from build123d import *

# Parameters (mm, degrees)
PAD_DEPTH       = 2
BOX002_W        = 44
BOX002_H        = 17
BOX002_DEPTH    = 78
SKETCH003_R     = 4.1
SKETCH003_R_2   = 2
SKETCH003_W     = 49.28004
SKETCH003_H     = 11.88092
POCKET003_DEPTH = 17.001
BOX001_W        = 65
BOX001_H        = 34
BOX001_DEPTH    = 5
BOX_W           = 5
BOX_H           = 34
BOX_DEPTH       = 46
SKETCH_R        = 2.05
POCKET_DEPTH    = 5
SKETCH001_R     = 5
SKETCH001_R_2   = 1.7
POCKET001_DEPTH = 5
SKETCH002_R     = 4.5
POCKET002_DEPTH = 5
SKETCH007_R     = 11.05
POCKET004_DEPTH = 17.001
SKETCH008_R     = 12
SKETCH008_R_2   = 10
PAD001_DEPTH    = 2
CHAMFER_SIZE    = 1
CHAMFER001_SIZE = 1.999


with BuildPart() as pad:
    # Sketch006 → Pad (new body)
    with BuildSketch(Plane.XZ.offset(2)):
        Polygon((-30, 51), (35, 51), (35, 46), (5, 0), (0, 0), (-30, 46), align=None)
    extrude(amount=PAD_DEPTH)


with BuildPart() as pocket003:
    # Box002 → Box002 (new body)
    with BuildSketch(Plane(origin=(-19.5, 15, 51), x_dir=(1, 0, 0), z_dir=(0, 0, 1))):
        with Locations((22, 8.5)):
            Rectangle(BOX002_W, BOX002_H)
    extrude(amount=BOX002_DEPTH)

    # Sketch003 → Pocket003 (cut, through all)
    with BuildSketch(Plane(origin=(-19.5, 15, 51), x_dir=(1, 0, 0), z_dir=(0, -1, 0))):
        with Locations((22, 6)):
            Circle(SKETCH003_R)
        with Locations((22, 63)):
            Circle(SKETCH003_R)
        with Locations((6.95, 19.45)):
            Circle(SKETCH003_R_2)
        with Locations((37.05, 19.45)):
            Circle(SKETCH003_R_2)
        with Locations((6.95, 49.55)):
            Circle(SKETCH003_R_2)
        with Locations((37.05, 49.55)):
            Circle(SKETCH003_R_2)
        with Locations((21.985447, 75.94046)):
            Rectangle(SKETCH003_W, SKETCH003_H)
    extrude(amount=-POCKET003_DEPTH, mode=Mode.SUBTRACT)


with BuildPart() as cubo001:
    # Box001 → Box001 (new body)
    with BuildSketch(Plane(origin=(-30, -2, 46), x_dir=(1, 0, 0), z_dir=(0, 0, 1))):
        with Locations((32.5, 17)):
            Rectangle(BOX001_W, BOX001_H)
    extrude(amount=BOX001_DEPTH)


with BuildPart() as chamfer001:
    # Box → Box (new body)
    with BuildSketch(Plane(origin=(0, -2, 0), x_dir=(1, 0, 0), z_dir=(0, 0, 1))):
        with Locations((2.5, 17)):
            Rectangle(BOX_W, BOX_H)
    extrude(amount=BOX_DEPTH)

    # Fusion: union Cubo001
    add(cubo001.part)

    # Sketch → Pocket (cut)
    with BuildSketch(Plane.XY.offset(51)):
        with Locations((-36.05, -7.05)):
            Circle(SKETCH_R)
        with Locations((28.95, 3.05)):
            Circle(SKETCH_R)
        with Locations((-55.15, -7.05)):
            Circle(SKETCH_R)
        with Locations((9.85, 3.05)):
            Circle(SKETCH_R)
        with Locations((-4.85, 3.05)):
            Circle(SKETCH_R)
        with Locations((-23.95, 3.05)):
            Circle(SKETCH_R)
        with Locations((-23.95, 26.95)):
            Circle(SKETCH_R)
        with Locations((-4.85, 26.95)):
            Circle(SKETCH_R)
        with Locations((9.85, 26.95)):
            Circle(SKETCH_R)
        with Locations((28.95, 26.95)):
            Circle(SKETCH_R)
    extrude(amount=-POCKET_DEPTH, mode=Mode.SUBTRACT)

    # Sketch001 → Pocket001 (cut)
    with BuildSketch(Plane.YZ.offset(5)):
        with Locations((15, 11)):
            Circle(SKETCH001_R)
        with Locations((15, 19.2)):
            Circle(SKETCH001_R_2)
        with Locations((23.2, 11)):
            Circle(SKETCH001_R_2)
        with Locations((15, 2.8)):
            Circle(SKETCH001_R_2)
        with Locations((6.8, 11)):
            Circle(SKETCH001_R_2)
    extrude(amount=-POCKET001_DEPTH, mode=Mode.SUBTRACT)

    # Sketch002 → Pocket002 (cut)
    with BuildSketch(Plane.YZ.offset(5)):
        with Locations((15, 34.8)):
            Circle(SKETCH002_R)
    extrude(amount=-POCKET002_DEPTH, mode=Mode.SUBTRACT)

    # Fusion001: union Pad, Pocket003
    add(pad.part)
    add(pocket003.part)

    # Sketch007 → Pocket004 (cut, through all)
    with BuildSketch(Plane.XZ.offset(-15)):
        with Locations((3.631613, 115.011309)):
            Circle(SKETCH007_R)
    extrude(amount=-POCKET004_DEPTH, mode=Mode.SUBTRACT)

    # Sketch008 → Pad001 (new body)
    with BuildSketch(Plane.XZ.offset(-15)):
        with Locations((2.5, 85.5)):
            Circle(SKETCH008_R)
        with Locations((2.5, 85.5)):
            Circle(SKETCH008_R_2, mode=Mode.SUBTRACT)
    extrude(amount=PAD001_DEPTH)

    # Chamfer
    chamfer_edges = [chamfer001.edges().sort_by_distance(p)[0] for p in [
        (-30, 32, 48.5),
    ]]
    chamfer(chamfer_edges, length=CHAMFER_SIZE)

    # Chamfer001
    chamfer001_edges = [chamfer001.edges().sort_by_distance(p)[0] for p in [
        (24.5, 32, 86),
    ]]
    chamfer(chamfer001_edges, length=CHAMFER001_SIZE)


solid = chamfer001.part
Can you work these out from the model? Positions are in its coordinate system, mm. A direction names the side the tool comes from. Give positions to 0.01 mm unless a question says otherwise; leave off trailing zeros. Loops run counter-clockwise (first coordinate to the right, second up) from the corner with the lowest first, then second, coordinate; pieces in that order, holes last. Notation, with made-up numbers: M 19,3 L 74,3 A21 cw 74,36 Z; hole C -21.5,77.5 d11. An arc over 180 degrees is marked long. One line per item, written item: value. Start each with the question number.
1) If we section it at C-C, the plane x = 17: Write out the boundary of the cut face in (y, z), and give its area (3 significant figures).
2) If we section it at B-B, the plane z = 100.55: Write out the boundary of the cut face in (x, y), and give its area (3 significant figures).
3) Thinking about a two-plate mould opening in Y: for faces 1 (the face through (-6.9, 3.1, 48.5)), 2 (the face through (3.3, 23.381, 103.966)), which applies, +Y half, -Y half, draft (parallel to the pull), parting line (faces both ways), or undercut?
4) If we section it at D-D, the plane z = 49: Give the number of separate pieces and of enclosed holes in the cut face, and give its area (3 significant figures).
5) If I drill on line 1 (Y direction, x = 9.85, z = 49.55); line 2 (Z direction, x = 17.55, y = 22); line 3 (Y direction, x = -23, z = 49), over which ranges is the centre line in solid material (lowest first)? Write a range as [from, to].
6) I'm going to push flat-ended pins straight in: pin 1 (5.5 mm diameter, centred on y = 15, z = 2.8, fed in from -X); pin 2 (6.5 mm diameter, centred on x = -12.55, z = 70.45, fed in from -Y); pin 3 (4.5 mm diameter, centred on x = 9.85, y = 3.05, fed in from -Z); pin 4 (3 mm diameter, centred on x = 17.55, z = 100.55, fed in from -Y). Where does each tip first touch, or does it pass through?
7) If we section it at A-A, the plane y = 23.2: Write out the boundary of the cut face in (x, z).
8) On a 3-axis mill with a long thin cutter (end or side, diameter ignored), from which of +Z, -Z, +X, -X, +Y, -Y can I reach the whole of each face in a straight line? I mean faces 3 (the face through (5, 15, 23)), 4 (the face through (2.535, 6.579, 12.686)), 5 (the face through (8.339, 4.435, 48.535)), 6 (the face through (24.5, 22, 86)), 7 (the face through (10, 27, 51)). Say none if no direction works.
Completed:
1. outline: M -4,18.4 L -2,18.4 L -2,46 L 32,46 L 32,68.53 L 15,68.53 L 15,51 L -4,51 Z; M 15,72.37 L 32,72.37 L 32,98.63 L 15,98.63 Z; M 15,102.47 L 32,102.47 L 32,121 L 15,121 Z
1. area: 1,290 mm^2
2. outline: M -19.5,15 L -14.55,15 L -14.55,32 L -19.5,32 Z; M -10.55,15 L 15.55,15 L 15.55,32 L -10.55,32 Z; M 19.55,15 L 24.5,15 L 24.5,30 L 22.5,32 L 19.55,32 Z
2. area: 610 mm^2
3. face 1: undercut
3. face 2: draft
4. separate pieces: 1
4. enclosed holes: 8
4. area: 2,230 mm^2
5. line 1: y = [-4, 1], [5.1, 24.9], [29, 32]
5. line 2: z = [46, 68.45], [72.45, 98.55], [102.55, 121]
5. line 3: y = [-4, 1.23], [4.87, 25.13], [28.77, 32]
6. pin 1: stops at x = 0
6. pin 2: stops at y = 15
6. pin 3: stops at z = 46
6. pin 4: passes through
7. outline: M -30,46 L 0,46 L 0,12.7 L 5,12.7 L 5,46 L 35,46 L 35,51 L 24.5,51 L 24.5,121 L 12.92,121 A11.05 cw long -5.65,121 L -19.5,121 L -19.5,51 L -30,51 Z; M 0,0 L 5,0 L 5,9.3 L 0,9.3 Z; hole C -12.55,70.45 d4; hole C -12.55,100.55 d4; hole C 2.5,57 d8.2; hole C 17.55,70.45 d4; hole C 17.55,100.55 d4
8. face 3: -Z, +X, +Y
8. face 4: +X, -X
8. face 5: +Z, -Z
8. face 6: +Z, +X, +Y, -Y
8. face 7: -Z
